The listing builds one solid part. Answer for the finished solid, in the listing's coordinates (mm). A direction names the side the tool comes from. Coordinates: 2 decimals unless noted, no trailing zeros. Write each loop counter-clockwise with the first axis right and the second up, starting at its lowest first coordinate (ties: lowest second). Pieces come first, ordered by that corner, then holes.
Autodesk Inventor part; units mm, degrees
ref_plane "YZ Plane" through (0, 0, 0) normal (1, 0, 0) x (0, 1, 0)
ref_plane "XZ Plane" through (0, 0, 0) normal (0, 1, 0) x (-1, 0, 0)
ref_plane "XY Plane" through (0, 0, 0) normal (0, 0, 1) x (1, 0, 0)
sketch "Sketch1" plane through (0, 0, 0) normal (0, 0, 1) x (1, 0, 0)
  line L0 (0, 0) -> (93, 0)
  line L1 (0, 12.15) -> (0, 27)
  line L2 (0, 27) -> (2, 27)
  line L3 (2, 27) -> (2, 62.5)
  line L4 (2, 62.5) -> (17.9, 62.5)
  line L5 (17.9, 62.5) -> (17.9, 27)
  line L6 (17.9, 27) -> (28.2, 16.7)
  line L7 (28.2, 16.7) -> (59.7364, 16.7)
  line L8 (59.7364, 16.7) -> (62, 13.75)
  line L9 (62, 13.75) -> (62, 12.15)
  line L10 (62, 12.15) -> (0, 12.15)
  point P0 (0, 19.575)
  dimension "d5" = 125
  dimension "d6" = 54
  dimension "d7" = 2
  dimension "d8" = 15.9
  dimension "d9" = 45
  dimension "d10" = 60
  dimension "d27" = 37.5
  dimension "d28" = 24.3
  dimension "d29" = 33.4
  dimension "d30" = 1.6
revolve "Revolution1" add sketch "Sketch1" angle 360 about axis through (0, 0, 0) along (1, 0, 0)
sketch "Sketch3" plane through (2, 0, 0) normal (-1, 0, 0) x (0, 0, 1)
  point P0 (0, 0)
  point P1 (0, 44.45)
  dimension "d16" = 44.45
hole "Hole1" at (2, 44.45, 0) direction (1, 0, 0) diameter 19.05 end up to surface
pattern_circular "Circular Pattern1" count 4 over 360 about axis through (9.95, 0, 0) along (1, 0, 0) of "Hole1"
properties part number "Flange 1 in" material "ASTM A105 Gr.B"
1. A tool of negligible diameter and unlimited length cuts with its end or side. For faces 1 (the cylindrical face through (1.01, -5.85, -26.36)), 2 (the cylindrical face through (10.061, -0.419, 34.934)), 3 (the cylindrical face through (44.189, 15.929, 5.016)), from which of +Z, -Z, +X, -X, +Y, -Y can it reach the whole face along a straight path? Write none if from no direction.
Results found:
face 1: -X
face 2: +X, -X
face 3: +X
2. Section C-C on z = -44.45 is taken. Give the vertices of the cut face in (x, y) (3 decimals).
Results found:
outline: (2, -43.937) - (17.9, -43.937) - (17.9, -9.525) - (2, -9.525) - close; (2, 9.525) - (17.9, 9.525) - (17.9, 43.937) - (2, 43.937) - close
3. Section B-B on x = 13.5 is taken. Give the vertices of the cut face in (y, z) (3 decimals), then the cut area to 3 significant figures.
Results found:
outline: circle Ø125 at (0, 0); hole circle Ø19.05 at (-44.45, 0); hole circle Ø24.3 at (0, 0); hole circle Ø19.05 at (0, -44.45); hole circle Ø19.05 at (0, 44.45); hole circle Ø19.05 at (44.45, 0)
area: 10,700 mm2
4. Flat-ended cylindrical pins translate along their axes: P1, Ø3, axis at y = -2, z = 31.5, coming from the -X side; P2, Ø4, axis at x = 35.5, z = -7.5, coming from the -Y side; P3, Ø8, axis at x = 12.5, y = -28.5, coming from the -Z side. Find the tip coordinate at first contact, or state that the pin passes through.
Results found:
P1: stops at x = 2
P2: stops at y = -15.77
P3: stops at z = -57.5
5. Section D-D on y = 41.5 is taken. Give the vertices of the cut face in (x, z), then the cut area to 3 significant figures.
Results found:
outline: (2, -46.73) - (17.9, -46.73) - (17.9, -9.06) - (2, -9.06) - close; (2, 9.06) - (17.9, 9.06) - (17.9, 46.73) - (2, 46.73) - close
area: 1,200 mm2
6. Find the intervals of material crossed by L1, parallel to Z at x = 10, y = 0 (3 decimals); L2, parallel to X at y = 22.5, z = 48; L3, parallel to Y at x = 5, z = 44, in increasing order.
Results found:
L1: z = -62.5 to -53.975, -34.925 to -12.15, 12.15 to 34.925, 53.975 to 62.5
L2: x = 2 to 17.9
L3: y = -44.39 to -9.51, 9.51 to 44.39
7. For a pull along Z with two mould halves and no side action, classify faces 4 (the flat face through (2, 27, -13)), 5 (the cylindrical face through (10.1, -53.9, -1.2)), 6 (the conical face through (61.86, -3.02, 13.6)), 7 (the cylindrical face through (10.1, 35, -1.2)) as pulls with the +Z half, pulls with the -Z half, needs draft (parallel to the pull), parting line crosses it, or undercut.
Results found:
face 4: needs draft
face 5: undercut
face 6: parting line crosses it
face 7: undercut
8. Section A-A on y = 0 is taken. Give the vertices of the cut face in (x, z) (3 decimals).
Results found:
outline: (0, -27) - (2, -27) - (2, -34.925) - (17.9, -34.925) - (17.9, -27) - (28.2, -16.7) - (59.736, -16.7) - (62, -13.75) - (62, -12.15) - (0, -12.15) - close; (0, 12.15) - (62, 12.15) - (62, 13.75) - (59.736, 16.7) - (28.2, 16.7) - (17.9, 27) - (17.9, 34.925) - (2, 34.925) - (2, 27) - (0, 27) - close; (2, -62.5) - (17.9, -62.5) - (17.9, -53.975) - (2, -53.975) - close; (2, 53.975) - (17.9, 53.975) - (17.9, 62.5) - (2, 62.5) - close
